Model file for the job. Use its own axes, mm. A direction names the side the tool comes from. Round coordinates to 2 decimals unless told otherwise and drop trailing zeros. Order: outer loops, then holes, each group sorted by start corner. A loop starts at its lowest first (then second) coordinate and runs counter-clockwise, first axis right, second up. Notation, with made-up numbers: (10.25, 81) -> (44.25, 81) arc R23 cw to (44.25, 102) -> close; hole circle Ø3 at (89.25, 38). An arc over 180 degrees is marked (long way). Answer as CSV lines item,"result".
```python
from build123d import *

# Parameters (mm, degrees)
SKETCH1_W           = 311.15
SKETCH1_H           = 488.95
BOSS_EXTRUDE1_DEPTH = 53.34
FILLET1_R           = 4
SHELL1_START        = -151.575
SHELL1_OUTLINE_W    = 49.34
SHELL1_OUTLINE_H    = 480.95
SHELL1_DEPTH        = 303.15
SKETCH2_R           = 12.67938946
CUT_EXTRUDE1_DEPTH  = 400.283738368


# Read off the part's stored shape, not the designer's step: Shell1
with BuildPart() as part:
    # Sketch1 → Boss-Extrude1 (new body)
    with BuildSketch(Plane(origin=(0, 0, 0), x_dir=(1, 0, 0), z_dir=(0, 1, 0))):
        Rectangle(SKETCH1_W, SKETCH1_H)
    extrude(amount=BOSS_EXTRUDE1_DEPTH)

    # Fillet1
    fillet1_edges = [part.edges().sort_by_distance(p)[0] for p in [
        (155.575, 53.34, 0),
        (0, 53.34, -244.475),
        (-155.575, 53.34, 0),
        (-155.575, 26.67, -244.475),
        (155.575, 26.67, -244.475),
        (155.575, 26.67, 244.475),
        (-155.575, 26.67, 244.475),
        (0, 53.34, 244.475),
    ]]
    fillet(fillet1_edges, radius=FILLET1_R)

    # Shell1 outline → Shell1 (cut)
    with BuildSketch(Plane.YZ.offset(SHELL1_START)):
        with Locations((24.67, 0)):
            Rectangle(SHELL1_OUTLINE_W, SHELL1_OUTLINE_H)
    extrude(amount=SHELL1_DEPTH, mode=Mode.SUBTRACT)

    # Sketch2 → Cut-Extrude1 (cut, through all)
    with BuildSketch(Plane(origin=(155.575, 0, 0), x_dir=(0, 0, -1), z_dir=(1, 0, 0))):
        with Locations((-209.55, 26.67)):
            Circle(SKETCH2_R)
        with Locations((209.55, 26.67)):
            Circle(SKETCH2_R)
    extrude(amount=-CUT_EXTRUDE1_DEPTH, mode=Mode.SUBTRACT)


solid = part.part
```
Q1. Saw through at C-C (x = 21). Write the cut outline in (y, z) (3 decimals), plus the area to 3 significant figures.
Checks:
outline,"(0, -244.475) -> (49.34, -244.475) arc R4 ccw to (53.34, -240.475) -> (53.34, 240.475) arc R4 ccw to (49.34, 244.475) -> (0, 244.475) -> (0, 240.475) -> (49.34, 240.475) -> (49.34, -240.475) -> (0, -240.475) -> close"
area,"2,340 mm²"
Q2. Flat gauge pin, fed straight in: pin 1 (1 mm diameter, centred on x = -77, z = -143.5, fed in from -Y). Where does the tip first touch, or does it go through?
Checks:
pin 1,"y = 49.34"
Q3. Saw through at A-A (z = -209.55). Write the cut outline in (x, y) (3 decimals).
Checks:
outline,"(-155.575, 0) -> (-151.575, 0) -> (-151.575, 13.991) -> (-155.575, 13.991) -> close; (-155.575, 39.349) -> (-151.575, 39.349) -> (-151.575, 49.34) -> (151.575, 49.34) -> (151.575, 39.349) -> (155.575, 39.349) -> (155.575, 49.34) arc R4 ccw to (151.575, 53.34) -> (-151.575, 53.34) arc R4 ccw to (-155.575, 49.34) -> close; (151.575, 0) -> (155.575, 0) -> (155.575, 13.991) -> (151.575, 13.991) -> close"
Q4. Mould opens along Y. For faces 1 (the flat face through (-2, 49.34, -3)), 2 (the cylindrical face through (153.6, 21.81, 197.84)), 3 (the flat face through (155.575, 24, 3)), 4 (the cylindrical face through (153.6, 21.81, -221.26)) say: +Y half, -Y half, draft (parallel to the pull), parting line (faces both ways), or undercut.
Checks:
face 1,"-Y half"
face 2,"undercut"
face 3,"draft"
face 4,"undercut"
Q5. Tool access for faces 5 (the flat face through (-2, 24, -240.475)), 6 (the flat face through (-155.575, 24, 3)): list every direction of +Z, -Z, +X, -X, +Y, -Y with a clear straight run to the whole face (end or side of a thin tool).
Checks:
face 5,"-Y"
face 6,"+Z, -Z, -X, +Y, -Y"
Q6. Wall check: L1, parallel to Z at x = 152, y = 26; L2, parallel to X at y = 11, z = -206 (3 decimals); L3, parallel to Z at x = -18.5, y = 13 (3 decimals). Give the ranges that are in metal, low to high. Write a range as [from, to].
Checks:
L1,"[-244.45, -222.21], [-196.89, 196.89], [222.21, 244.45]"
L2,"[-155.575, -151.575], [151.575, 155.575]"
L3,"[-244.475, -240.475], [240.475, 244.475]"
Q7. Saw through at B-B (y = 26.67). Write the cut outline in (x, z) (3 decimals), plus the area to 3 significant figures.
Checks:
outline,"(-155.575, -240.475) arc R4 ccw to (-151.575, -244.475) -> (151.575, -244.475) arc R4 ccw to (155.575, -240.475) -> (155.575, -222.229) -> (151.575, -222.229) -> (151.575, -240.475) -> (-151.575, -240.475) -> (-151.575, -222.229) -> (-155.575, -222.229) -> close; (-155.575, -196.871) -> (-151.575, -196.871) -> (-151.575, 196.871) -> (-155.575, 196.871) -> close; (-155.575, 222.229) -> (-151.575, 222.229) -> (-151.575, 240.475) -> (151.575, 240.475) -> (151.575, 222.229) -> (155.575, 222.229) -> (155.575, 240.475) arc R4 ccw to (151.575, 244.475) -> (-151.575, 244.475) arc R4 ccw to (-155.575, 240.475) -> close; (151.575, -196.871) -> (155.575, -196.871) -> (155.575, 196.871) -> (151.575, 196.871) -> close"
area,"5,920 mm²"
Q8. Saw through at D-D (z = 180). Write the cut outline in (x, y) (3 decimals), plus the area to 3 significant figures.
Checks:
outline,"(-155.575, 0) -> (-151.575, 0) -> (-151.575, 49.34) -> (151.575, 49.34) -> (151.575, 0) -> (155.575, 0) -> (155.575, 49.34) arc R4 ccw to (151.575, 53.34) -> (-151.575, 53.34) arc R4 ccw to (-155.575, 49.34) -> close"
area,"1,630 mm²"
